Verification items for this drawing (mm, ordinates from the low corner). A direction names the side the tool comes from. Coordinates: 2 decimals unless noted, no trailing zeros. Order: outer loops, then holes, each group sorted by start corner. A loop starts at its lowest first (then second) coordinate and runs counter-clockwise, first axis right, second up. Notation, with made-up numbers: M -38,-26 L 17,-26 A20 ccw 17,-13 Z; hole C 59,10.5 d5. An arc over 180 degrees is marked long. Answer as a JSON object with one key per item and string values. Group by question number.
(1) Cross-section at B-B (y = 13). Enter the section's corners in (x, z).
(2) Access from +Z, -Z, +X, -X, +Y, -Y to the whole of each face (thin tool, end or side, straight path). Record for the marked faces 1, 2 and 3.
(3) Cross-section at D-D (z = 19). Enter the section's corners in (x, y) (1 decimal), plus the area to 3 significant figures.
(4) Cross-section at C-C (z = 72.5). Enter the section's corners in (x, y) (1 decimal).
(5) Cross-section at A-A (x = 15). Enter the section's corners in (y, z) (1 decimal).
(6) Material ranges on line 1 (Y direction, x = 18.5, z = 205) (1 decimal); line 2 (Z direction, x = 3.5, y = 15); line 3 (Y direction, x = 18, z = 224) (1 decimal), recorded low to high.
(7) Gauge pin test, flat ends, axial feed: pin 1 Ø6 at (y, z) = (20.5, 119.5) entering from -X (1 decimal); pin 2 Ø5 at (y, z) = (6.5, 103) entering from -X (1 decimal); pin 3 Ø6 at (x, z) = (11.5, 49) entering from +Y. Record the tip position at first contact, or that the pin passes through.
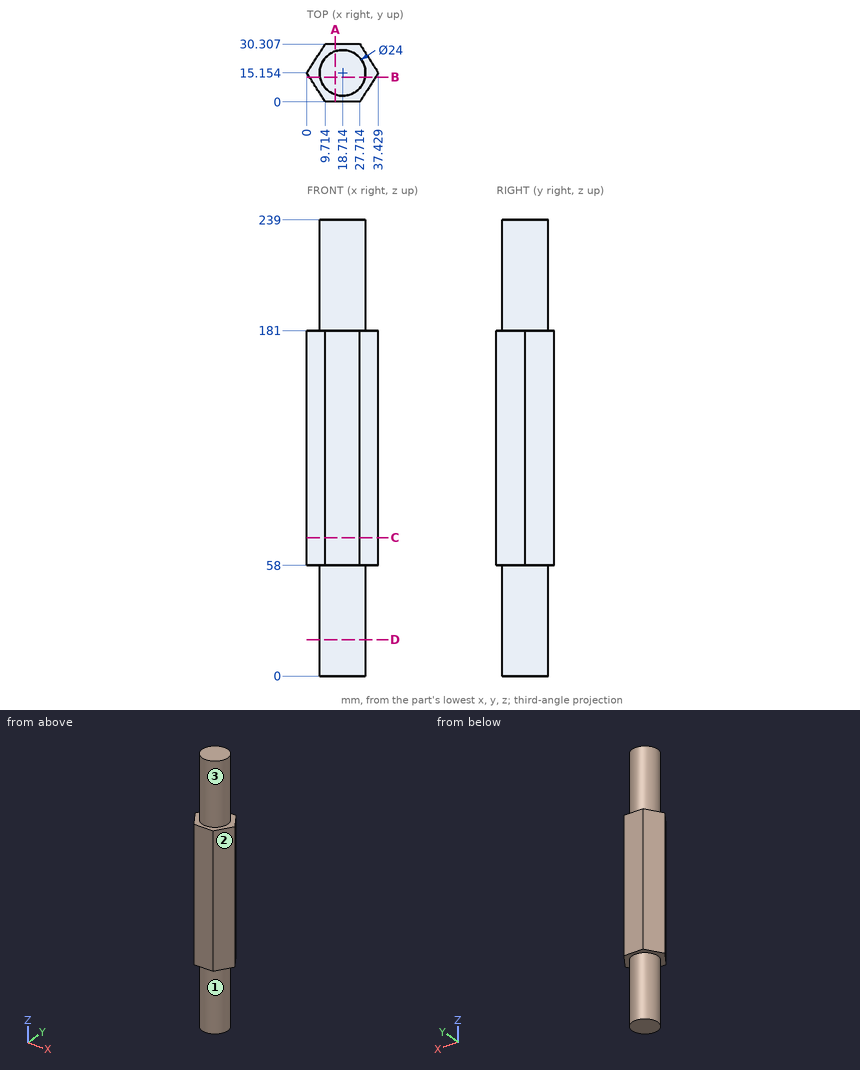
Taken from the geometry:
{
 "1": {"outline": "M 1.38,58 L 6.91,58 L 6.91,0 L 30.52,0 L 30.52,58 L 36.05,58 L 36.05,181 L 30.52,181 L 30.52,239 L 6.91,239 L 6.91,181 L 1.38,181 Z"},
 "2": {"face 1": "-Z", "face 2": "+Z, -Z, +X, -Y", "face 3": "+Z"},
 "3": {"outline": "C 18.7,15.2 d24", "area": "452 mm²"},
 "4": {"outline": "M 0,15.2 L 9.7,0 L 27.7,0 L 37.4,15.2 L 27.7,30.3 L 9.7,30.3 Z"},
 "5": {"outline": "M 0,58 L 3.7,58 L 3.7,0 L 26.6,0 L 26.6,58 L 30.3,58 L 30.3,181 L 26.6,181 L 26.6,239 L 3.7,239 L 3.7,181 L 0,181 Z"},
 "6": {"line 1": "y = 3.2 to 27.2", "line 2": "z = 58 to 181", "line 3": "y = 3.2 to 27.1"},
 "7": {"pin 1": "stops at x = 1.5", "pin 2": "stops at x = 3.9", "pin 3": "stops at y = 26.39"}
}
